Autodesk Fusion 360 part; units mm, degrees
sketch "Sketch1" plane through (0, 0, 0) normal (0, 1, 0) x (1, 0, 0)
  circle A0 centre (0, 0) radius 14 construction
  circle A1 centre (0, 0) radius 48 construction
  circle A2 centre (0, 0) radius 58 construction
  circle A3 centre (0, 0) radius 68 construction
  line L0 (0, 0) -> (0, 52) construction
  line L1 (-9.7468, 47) -> (-49.1426, 47) construction
  line L2 (-35.0918, 32.75) -> (-59.5939, 32.75) construction
  line L3 (-39.023, 27.95) -> (-61.9903, 27.95) construction
  line L4 (-42.7385, -21.85) -> (-64.3939, -21.85) construction
  circle A4 centre (-50.3158, -28.85) radius 1.5
  circle A5 centre (-42.1187, 39.875) radius 1.5
  line L5 (-55.3158, -21.85) -> (-55.3158, -28.85)
  line L6 (-50.3158, -33.85) -> (-22.1187, -33.85)
  line L7 (-22.1187, -21.85) -> (-22.1187, 27.95)
  line L8 (-27.1187, 44.875) -> (-47.1187, 44.875)
  line L9 (-52.1187, -21.85) -> (-55.3158, -21.85)
  line L10 (-30.1187, 27.95) -> (-40.1187, 27.95)
  arc A6 (-50.3158, -33.85) -> (-55.3158, -28.85) centre (-50.3158, -28.85) ccw construction
  arc A7 (-55.3158, -28.85) -> (-50.3158, -33.85) centre (-50.3158, -28.85) ccw
  line L11 (-55.3158, -33.85) -> (-50.3158, -33.85) construction
  line L12 (-55.3158, -28.85) -> (-55.3158, -33.85) construction
  line L13 (-22.1187, -21.85) -> (-17.1187, -21.85)
  line L14 (-17.1187, -21.85) -> (-17.1187, -28.85)
  line L15 (-22.1187, -33.85) -> (-17.1187, -33.85) construction
  line L16 (-17.1187, -28.85) -> (-17.1187, -33.85) construction
  arc A8 (-17.1187, -28.85) -> (-22.1187, -33.85) centre (-22.1187, -28.85) ccw construction
  arc A9 (-22.1187, -33.85) -> (-17.1187, -28.85) centre (-22.1187, -28.85) ccw
  line L17 (-65.8278, -17.05) -> (-44.8698, -17.05) construction
  line L18 (-40.1187, -21.85) -> (-30.1187, -21.85)
  line L19 (-30.1187, -21.85) -> (-30.1187, -26.65)
  line L20 (-30.1187, -26.65) -> (-40.1187, -26.65)
  line L21 (-40.1187, -26.65) -> (-40.1187, -21.85)
  line L22 (-40.1187, 27.95) -> (-40.1187, 23.15)
  line L23 (-40.1187, 23.15) -> (-30.1187, 23.15)
  line L24 (-30.1187, 23.15) -> (-30.1187, 27.95)
  line L25 (-30.1187, -21.85) -> (-22.1187, -21.85) construction
  line L26 (-52.1187, 27.95) -> (-47.1187, 27.95)
  line L27 (-47.1187, 27.95) -> (-47.1187, 44.875)
  line L28 (-22.1187, 27.95) -> (-27.1187, 27.95)
  line L29 (-27.1187, 27.95) -> (-27.1187, 44.875)
  line L30 (-27.1187, 27.95) -> (-30.1187, 27.95) construction
  line L31 (-52.1187, 27.95) -> (-52.1187, -21.85)
  point P0 (0, 14)
  point P1 (-42.1187, 39.875)
  point P2 (-50.3158, -28.85)
  dimension "d1" = 28
  dimension "d2" = 96
  dimension "d3" = 116
  dimension "d4" = 136
  dimension "d5" = 38
  dimension "d6" = 5
  dimension "d7" = 19.25
  dimension "d8" = 4.8
  dimension "d11" = 7
  dimension "d12" = 7.125
  dimension "d13" = 3
  dimension "d14" = 3
  dimension "d15" = 10
  dimension "d24" = 5
  dimension "d27" = 5
  dimension "d28" = 10
  dimension "d29" = 4.8
  dimension "d30" = 45
  dimension "d31" = 10
  dimension "d32" = 4.8
  dimension "d34" = 8
  dimension "d35" = 4.8
  dimension "d36" = 10
  dimension "d37" = 8
  dimension "d38" = 5
  dimension "d39" = 5
  dimension "d40" = 5
  dimension "d43" = 12
extrude "Extrude1" add sketch "Sketch1" along normal blind 4.8
fillet "Fillet1" radius 2 4 edges at (-37.1187, 0, -44.875) (-47.1187, 2.4, -44.875) (-37.1187, 4.8, -44.875) (-27.1187, 2.4, -44.875)
fillet "Fillet2" radius 2 1 edges at (-52.1187, 4.8, -3.05)
For this review, take the finished solid that the model builds, in its own axes (mm). A direction names the side the tool comes from. Coordinates: 2 decimals unless noted, no trailing zeros. Loops run counter-clockwise (first coordinate to the right, second up) from the corner with the lowest first, then second, coordinate; pieces in that order, holes last. Notation, with made-up numbers: (24, 29) -> (75, 29) arc R28 cw to (75, 58) -> close; hole circle Ø6 at (80, 48). An arc over 180 degrees is marked (long way). Write each question's results on one line, items separated by ' | '.
Q1. Mouldability with a two-part tool opening along X and no side actions: class faces 1 (the cylindrical face through (-51.517, 4.23, -2.701)), 2 (the cylindrical face through (-37.259, 4.23, -44.274)), 3 (the flat face through (-30.119, 2, -26)) as +X half, -X half, draft (parallel to the pull), parting line (faces both ways), or undercut.
Taken from the geometry:
face 1: -X half | face 2: draft | face 3: undercut
Q2. Add section A-A, the plane z = 25.5. State the section outline as (x, y) points, then the cut area to 3 significant figures.
Taken from the geometry:
outline: (-55.32, 0) -> (-40.12, 0) -> (-40.12, 4.8) -> (-55.32, 4.8) -> close; (-30.12, 0) -> (-17.12, 0) -> (-17.12, 4.8) -> (-30.12, 4.8) -> close | area: 135 mm²
Q3. Add section B-B, the plane y = 0.8. State the section outline as (x, z) points (3 decimals).
Taken from the geometry:
outline: (-55.316, 21.85) -> (-52.119, 21.85) -> (-52.119, -27.95) -> (-47.119, -27.95) -> (-47.119, -42.875) arc R2 ccw to (-46.319, -44.475) -> (-27.919, -44.475) arc R2 ccw to (-27.119, -42.875) -> (-27.119, -27.95) -> (-22.119, -27.95) -> (-22.119, 21.85) -> (-17.119, 21.85) -> (-17.119, 28.85) arc R5 ccw to (-22.119, 33.85) -> (-50.316, 33.85) arc R5 ccw to (-55.316, 28.85) -> close; hole circle Ø3 at (-50.316, 28.85); hole circle Ø3 at (-42.119, -39.875); hole (-40.119, -27.95) -> (-30.119, -27.95) -> (-30.119, -23.15) -> (-40.119, -23.15) -> close; hole (-40.119, 21.85) -> (-30.119, 21.85) -> (-30.119, 26.65) -> (-40.119, 26.65) -> close
Q4. To check wall thickness, follow line 1 along Z through (x, y) = (-31, 1.15); line 2 along X through (y, z) = (2.65, -4); line 3 along X through (y, z) = (2, -35.5). State the ranges of each line that lie inside material, in increasing order. Write a range as [from, to].
Taken from the geometry:
line 1: [-44.69, -27.95], [-23.15, 21.85], [26.65, 33.85] | line 2: [-52.12, -22.12] | line 3: [-47.12, -27.12]
Q5. Add section C-C, the plane z = 15.5. State the section outline as (x, y) points, then the cut area to 3 significant figures.
Taken from the geometry:
outline: (-52.12, 0) -> (-22.12, 0) -> (-22.12, 4.8) -> (-50.12, 4.8) arc R2 ccw to (-52.12, 2.8) -> close | area: 143 mm²
Q6. For pin 1 Ø0.8 at (y, z) = (1, -1) entering from -X; pin 2 Ø1.4 at (x, y) = (-20, 3) entering from -Z; pin 3 Ø2.5 at (y, z) = (2.5, -35) entering from +X, all flat-tipped, find the tip position at first contact; note any pin that passes through.
Taken from the geometry:
pin 1: x = -52.12 | pin 2: z = 21.85 | pin 3: x = -27.12
Q7. Machinability: for faces 4 (the flat face through (-27.119, 2, -35)), 5 (the flat face through (-55.316, 2, 25)), 6 (the flat face through (-47.119, 2, -35)), 7 (the cylindrical face through (-53.812, 2.366, 32.424)), 8 (the flat face through (-40.119, 2, 24)), which of the approach directions +Z, -Z, +X, -X, +Y, -Y give a long, thin tool a straight path to every point of the face, cutting with its end or side? Answer none if there is none.
Taken from the geometry:
face 4: -Z, +X, +Y, -Y | face 5: +Z, -Z, -X, +Y, -Y | face 6: -Z, -X, +Y, -Y | face 7: +Z, -X, +Y, -Y | face 8: +Y, -Y
Q8. Add section D-D, the plane x = -26. State the section outline as (y, z) points.
Taken from the geometry:
outline: (0, -27.95) -> (4.8, -27.95) -> (4.8, 33.85) -> (0, 33.85) -> close
